```python
from build123d import *

# Parameters (mm, degrees)
ESQUISSE1_W        = 86.7
ESQUISSE1_H        = 86.7
ESQUISSE1_W_2      = 16.7
ESQUISSE1_H_2      = 16.7
BOSS_EXTRU_1_DEPTH = 3.5
ESQUISSE2_W        = 86.7
ESQUISSE2_H        = 86.7
BOSS_EXTRU_2_DEPTH = 1


with BuildPart() as part:
    # Esquisse1 → Boss.-Extru.1 (new body)
    with BuildSketch(Plane(origin=(0, 0, 0), x_dir=(1, 0, 0), z_dir=(0, 1, 0))):
        with Locations((43.35, 43.35)):
            Rectangle(ESQUISSE1_W, ESQUISSE1_H)
        with Locations((43.35, 18.35)):
            Rectangle(ESQUISSE1_W_2, ESQUISSE1_H_2, mode=Mode.SUBTRACT)
        with Locations((18.35, 18.35)):
            Rectangle(ESQUISSE1_W_2, ESQUISSE1_H_2, mode=Mode.SUBTRACT)
        with Locations((68.35, 18.35)):
            Rectangle(ESQUISSE1_W_2, ESQUISSE1_H_2, mode=Mode.SUBTRACT)
        with Locations((43.35, 43.35)):
            Rectangle(ESQUISSE1_W_2, ESQUISSE1_H_2, mode=Mode.SUBTRACT)
        with Locations((68.35, 43.35)):
            Rectangle(ESQUISSE1_W_2, ESQUISSE1_H_2, mode=Mode.SUBTRACT)
        with Locations((43.35, 68.35)):
            Rectangle(ESQUISSE1_W_2, ESQUISSE1_H_2, mode=Mode.SUBTRACT)
        with Locations((68.35, 68.35)):
            Rectangle(ESQUISSE1_W_2, ESQUISSE1_H_2, mode=Mode.SUBTRACT)
        with Locations((18.35, 43.35)):
            Rectangle(ESQUISSE1_W_2, ESQUISSE1_H_2, mode=Mode.SUBTRACT)
        with Locations((18.35, 68.35)):
            Rectangle(ESQUISSE1_W_2, ESQUISSE1_H_2, mode=Mode.SUBTRACT)
    extrude(amount=BOSS_EXTRU_1_DEPTH)

    # Esquisse2 → Boss.-Extru.2 (add)
    with BuildSketch(Plane.XZ):
        with Locations((43.35, -43.35)):
            Rectangle(ESQUISSE2_W, ESQUISSE2_H)
    extrude(amount=BOSS_EXTRU_2_DEPTH)


solid = part.part
```
For this review, take the finished solid that the model builds, in its own axes (mm). Give positions to 0.01 mm unless a question says otherwise; leave off trailing zeros. Write each loop counter-clockwise with the first axis right and the second up, starting at its lowest first coordinate (ties: lowest second). Pieces come first, ordered by that corner, then holes. Notation, with made-up numbers: M 36.25,6 L 48.25,6 A24 ccw 48.25,29 Z; hole C 35.25,36.25 d9. An arc over 180 degrees is marked long. One line per item, written item: value.
1) Take a section at A-A, the plane z = -43. Write out the cut boundary in (x, y), then the cut area to 3 significant figures.
Results are:
outline: M 0,-1 L 86.7,-1 L 86.7,3.5 L 76.7,3.5 L 76.7,0 L 60,0 L 60,3.5 L 51.7,3.5 L 51.7,0 L 35,0 L 35,3.5 L 26.7,3.5 L 26.7,0 L 10,0 L 10,3.5 L 0,3.5 Z
area: 215 mm²
2) Take a section at B-B, the plane x = 47. Write out the cut boundary in (y, z).
Results are:
outline: M -1,-86.7 L 3.5,-86.7 L 3.5,-76.7 L 0,-76.7 L 0,-60 L 3.5,-60 L 3.5,-51.7 L 0,-51.7 L 0,-35 L 3.5,-35 L 3.5,-26.7 L 0,-26.7 L 0,-10 L 3.5,-10 L 3.5,0 L -1,0 Z
3) The part is to be moulded in two halves that separate along X. For faces 1 (the flat face through (0, 1, -44)), 2 (the flat face through (68, 0, -43)), say which applies: +X half, -X half, draft (parallel to the pull), parting line (faces both ways), or undercut.
Results are:
face 1: -X half
face 2: undercut
4) Take a section at C-C, the plane y = 2.3. Count the separate pieces of the cut face and the enclosed holes in it, then the cut area to 3 significant figures.
Results are:
separate pieces: 1
enclosed holes: 9
area: 5,010 mm²
5) For line 1 (X direction, y = 0.3, z = -19.5); line 2 (Z direction, x = 39, y = 1.65); line 3 (Y direction, x = 35.5, z = -22), list the stretches that pass through material, from the lowest coordinate up. Write a range as from..to.
Results are:
line 1: x = 0..10, 26.7..35, 51.7..60, 76.7..86.7
line 2: z = -86.7..-76.7, -60..-51.7, -35..-26.7, -10..0
line 3: y = -1..0
6) For P1, Ø3, axis at x = 49, z = -13, coming from the +Y side, flat-tipped, find the tip position at first contact; note if it passes through.
Results are:
P1: stops at y = 0
